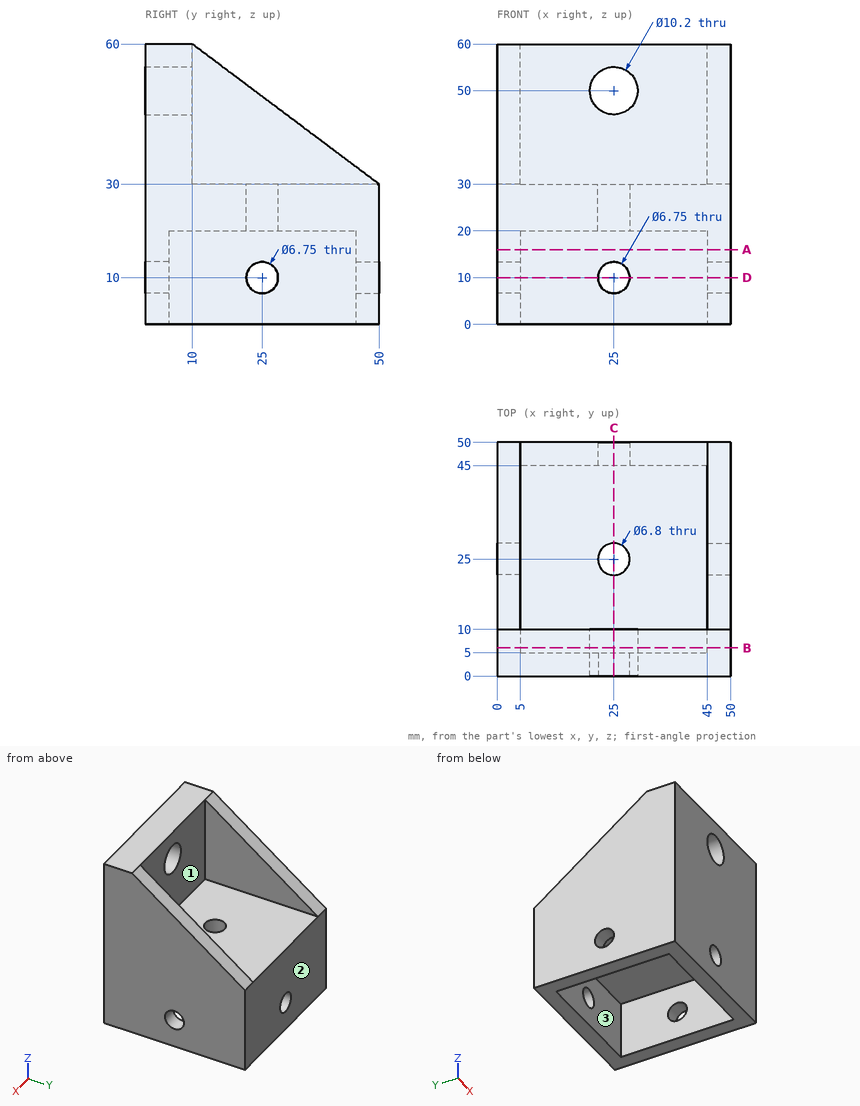
Geometry: see drawing. Coordinates: mm, zero at the bounding-box minimum. A direction names the side the tool comes from. Give positions to 0.01 mm unless a question says otherwise; leave off trailing zeros. Order: outer loops, then holes, each group sorted by start corner. A loop starts at its lowest first (then second) coordinate and runs counter-clockwise, first axis right, second up. Notation, with made-up numbers: (-27, 84.5) -> (32, 84.5) arc R13 cw to (32, 88.5) -> close; hole circle Ø4 at (-31.5, 37.5). An arc over 180 degrees is marked (long way). Write each question's results on one line, items separated by ' | '. Start each with the question number.
1) Section B-B (y = 6). Return loops of the section in (x, z), then the cut area to 3 significant figures.
2) Line query: line 1 (Z direction, x = 25, y = 3) (3 decimals); line 2 (Z direction, x = 25, y = 6); line 3 (Y direction, x = 40, z = 14.5). Output: solid intervals per line, ascending. Write a range as from..to.
3) Section A-A (z = 16). Return loops of the section in (x, y), then the cut area to 3 significant figures.
4) Section D-D (z = 10). Return loops of the section in (x, y) (3 decimals).
5) Section C-C (x = 25). Return loops of the section in (y, z) (3 decimals), then the cut area to 4 significant figures.
6) First-contact query: pin 1 (1.5 mm diameter, centred on x = 40, z = 47, fed in from +Y); pin 2 (9 mm diameter, centred on x = 25, y = 25, fed in from -Z); pin 3 (4 mm diameter, centred on x = 25, z = 10, fed in from -Y). Flat tips, straight axial feed; report the tip coordinate or a pass-through.
7) Set-up query: the marked faces 1, 2 and 3. Return all of +Z, -Z, +X, -X, +Y, -Y with unobstructed straight access to the full face (end or side cutting, diameter ignored); none if empty.
Calculated:
1) outline: (0, 0) -> (5, 0) -> (5, 20) -> (45, 20) -> (45, 0) -> (50, 0) -> (50, 60) -> (0, 60) -> close; hole circle Ø10.2 at (25, 50) | area: 2,120 mm2
2) line 1: 0..6.625, 13.375..44.9, 55.1..60 | line 2: 20..44.9, 55.1..60 | line 3: 0..5, 45..50
3) outline: (0, 0) -> (50, 0) -> (50, 50) -> (0, 50) -> close; hole (5, 5) -> (45, 5) -> (45, 45) -> (5, 45) -> close | area: 900 mm2
4) outline: (0, 0) -> (21.625, 0) -> (21.625, 5) -> (5, 5) -> (5, 21.625) -> (0, 21.625) -> close; (0, 28.375) -> (5, 28.375) -> (5, 45) -> (21.625, 45) -> (21.625, 50) -> (0, 50) -> close; (28.375, 0) -> (50, 0) -> (50, 21.625) -> (45, 21.625) -> (45, 5) -> (28.375, 5) -> close; (28.375, 45) -> (45, 45) -> (45, 28.375) -> (50, 28.375) -> (50, 50) -> (28.375, 50) -> close
5) outline: (0, 0) -> (5, 0) -> (5, 6.625) -> (0, 6.625) -> close; (0, 13.375) -> (5, 13.375) -> (5, 20) -> (21.6, 20) -> (21.6, 30) -> (10, 30) -> (10, 44.9) -> (0, 44.9) -> close; (0, 55.1) -> (10, 55.1) -> (10, 60) -> (0, 60) -> close; (28.4, 20) -> (45, 20) -> (45, 13.375) -> (50, 13.375) -> (50, 30) -> (28.4, 30) -> close; (45, 0) -> (50, 0) -> (50, 6.625) -> (45, 6.625) -> close | area: 762.5 mm2
6) pin 1: y = 10 | pin 2: z = 20 | pin 3: through
7) face 1: +Z, +Y | face 2: +Z, -Z, +X, -X, +Y | face 3: -Z
